```python
from build123d import *

# Parameters (mm, degrees)
F1_DEPTH = 25
F1_TAPER = -3
F2_R     = 12.5
F3_DEPTH = 50
F4_R     = 5.7994178108
F5_DEPTH = 50
F7_DEPTH = 10


# Not quite as in the source:
# - a feature names something its author has since deleted; it is built from what else it names


with BuildPart() as f1:
    # F0 (on Front) → F1 (new body)
    with BuildSketch(Plane.XZ):
        with BuildLine():
            Line((4.8843180895, 24.5182266243), (0, 25))
            ThreePointArc((0, 25), (-24.9682800601, -1.2589641933), (2.5147336452, -24.8732007328))
            ThreePointArc((2.5147336452, -24.8732007328), (18.5454622635, -16.7650180267), (25, 0))
            ThreePointArc((25, 0), (19.3275444927, 15.8570496588), (4.8843180895, 24.5182266243))
        make_face()
        with BuildLine():
            ThreePointArc((4.8843180895, 24.5182266243), (2.4540104311, 24.8792651178), (0, 25))
            Line((0, 25), (4.8843180895, 24.5182266243))
        make_face()
        with BuildLine():
            ThreePointArc((25, 0), (18.5454622635, -16.7650180267), (2.5147336452, -24.8732007328))
            Line((2.5147336452, -24.8732007328), (51.7188404795, -19.8985605862))
            ThreePointArc((51.7188404795, -19.8985605862), (29.7070684597, -0.0244101143), (51.6702619082, 19.9034120943))
            Line((51.6702619082, 19.9034120943), (4.8843180895, 24.5182266243))
            ThreePointArc((4.8843180895, 24.5182266243), (19.3275444927, 15.8570496588), (25, 0))
        make_face()
        with BuildLine():
            ThreePointArc((51.6702619082, 19.9034120943), (29.7070684597, -0.0244101143), (51.7188404795, -19.8985605862))
            ThreePointArc((51.7188404795, -19.8985605862), (64.5434233741, -13.4120144213), (69.7070535633, 0))
            ThreePointArc((69.7070535633, 0), (64.5270428835, 13.430112306), (51.6702619082, 19.9034120943))
        make_face()
    extrude(amount=F1_DEPTH, taper=F1_TAPER)

    # F2 (on Front) → F3 (join)
    with BuildSketch(Plane.XZ):
        Circle(F2_R)
        with Locations((50, 0)):
            Circle(F2_R)
    extrude(amount=F3_DEPTH)

    # F4 (on Front) → F5 (cut)
    with BuildSketch(Plane.XZ):
        with Locations((49.772053957, 0)):
            Circle(F4_R)
    extrude(amount=F5_DEPTH, mode=Mode.SUBTRACT)

    # F6 (on Front) → F7 (join)
    with BuildSketch(Plane.XZ):
        Polygon((-0.0836669881, -5.4505592747), (4.6784893026, -2.7977373745), (4.7621562908, 2.6528219002), (0.0836669881, 5.4505592747), (-4.6784893026, 2.7977373745), (-4.7621562908, -2.6528219002), align=None)
    extrude(amount=-F7_DEPTH)


solid = f1.part
```
Can you work these out from the model? Positions are in its coordinate system, mm. A direction names the side the tool comes from. Coordinates: 2 decimals unless noted, no trailing zeros. Loops run counter-clockwise (first coordinate to the right, second up) from the corner with the lowest first, then second, coordinate; pieces in that order, holes last. Notation, with made-up numbers: (41, 59) - (93, 59) arc R13 cw to (93, 68) - close; hole circle Ø1 at (20.5, 47). An arc over 180 degrees is marked (long way). Answer as CSV lines item,"result". Start each with the question number.
1) Suppose I cut it at A-A (y = -30). Please give me the cut outline in (x, z).
2) Which directions (+Z, -Z, +X, -X, +Y, -Y) give clear straight access to the entire face, cutting with the end or side of a thin tool? Please do faces 5 (the flat face through (2.264, 4.93, -4.143)), 6 (the flat face through (0, -50, 0)), 7 (the flat face through (-2.264, 4.93, 4.143)), 8 (the flat face through (-2.46, 4.93, -4.03)), 9 (the flat face through (22, -25, 0)).
3) For pin 1 (2 mm diameter, centred on x = 46, z = 20, fed in from +Y); pin 2 (4 mm diameter, centred on y = -42.5, z = 11.5, fed in from +X); pin 3 (10 mm diameter, centred on y = -7.5, z = 17.5, fed in from +X); pin 4 (7 mm diameter, centred on x = 49.77, z = 0, fed in from +Y), each with a flat end and sliding along its axis, tell me the tip position at first contact or that it passes through.
4) Thinking about a two-plate mould opening in Z: for faces 1 (the cylindrical face through (55.13, -24.65, -2.22)), 2 (the cylindrical face through (37.512, -37.325, 0.55)), 3 (the flat face through (2.46, 4.93, 4.03)), 4 (the conical face through (64.893, -12.675, -14.014)), which applies, pulls with the +Z half, pulls with the -Z half, needs draft (parallel to the pull), parting line crosses it, or undercut?
5) Suppose I cut it at B-B (y = 3). Please give me the cut outline in (x, z).
6) I need wall thicknesses on line 1 (Y direction, x = 45.5, z = 16.5); line 2 (Z direction, x = 50.5, y = -29); line 3 (Y direction, x = 47, z = 12). Which ranges of each line are inside material? Lowest first, please. Write a range as from..to.
Check result:
1,outline,"circle Ø25 at (0, 0); circle Ø25 at (50, 0); hole circle Ø11.6 at (49.77, 0)"
2,face 5,"-Z, +X, +Y"
2,face 6,"+Z, -Z, +X, -X, -Y"
2,face 7,"+Z, -X, +Y"
2,face 8,"-Z, -X, +Y"
2,face 9,"-Y"
3,pin 1,"stops at y = 0"
3,pin 2,"stops at x = 58.12"
3,pin 3,"stops at x = 65.83"
3,pin 4,"passes through"
4,face 1,"undercut"
4,face 2,"parting line crosses it"
4,face 3,"pulls with the +Z half"
4,face 4,"pulls with the -Z half"
5,outline,"(-4.76, -2.65) - (-0.08, -5.45) - (4.68, -2.8) - (4.76, 2.65) - (0.08, 5.45) - (-4.68, 2.8) - close"
6,line 1,"y = -25..0"
6,line 2,"z = -12.49..-5.75, 5.75..12.49"
6,line 3,"y = -50..0"
